from build123d import *

# Parameters (mm, degrees)
F0_R      = 6
F1_DEPTH  = 30
F2_R      = 2.75
F3_DEPTH  = 30.001
F8_R      = 5
F8_R_2    = 1.6
F9_DEPTH  = 2
F12_W     = 4
F12_H     = 30
F13_DEPTH = 3


with BuildPart() as f1:
    # F0 (on Front) → F1 (new body)
    with BuildSketch(Plane.XZ):
        Circle(F0_R)
    extrude(amount=F1_DEPTH)

    # F2 (on face) → F3 (cut, through all)
    with BuildSketch(Plane.XZ.offset(30)):
        Circle(F2_R)
    extrude(amount=-F3_DEPTH, mode=Mode.SUBTRACT)

    # F8 (on face) → F9 (join)
    with BuildSketch(Plane.XZ.offset(30)):
        Circle(F8_R)
        Circle(F8_R_2, mode=Mode.SUBTRACT)
    extrude(amount=-F9_DEPTH)

    # F12 (on offset) → F13 (cut)
    with BuildSketch(Plane.XY.offset(4)):
        with Locations((0, -15)):
            Rectangle(F12_W, F12_H)
    extrude(amount=F13_DEPTH, mode=Mode.SUBTRACT)


solid = f1.part
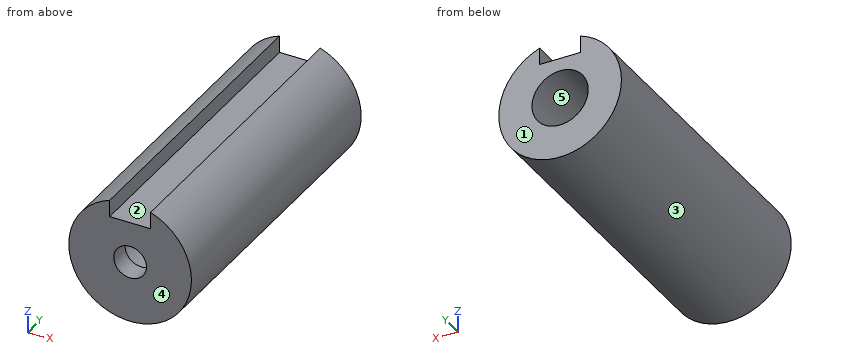
Part model, mm, in its own coordinate system. Face numbers are marked on the shaded views. A direction names the side the tool comes from. Round coordinates to 2 decimals unless told otherwise and drop trailing zeros. Write each loop counter-clockwise with the first axis right and the second up, starting at its lowest first coordinate (ties: lowest second). Pieces come first, ordered by that corner, then holes. Notation, with made-up numbers: M 34,-30.75 L 61,-30.75 A13 ccw 61,-11.75 Z; hole C 20,49 d6. An arc over 180 degrees is marked long. Return JSON: item names as keys, results as strings. Group by question number.
(1) Saw through at A-A on x = 0. Write the cut outline in (y, z), then the cut area to 3 significant figures.
(2) Saw through at B-B on z = 0. Write the cut outline in (x, y), then the cut area to 3 significant figures.
(3) Two-plate mould, pull along X, no slides. Class the marked faces 3, 4 and 5: +X half, -X half, draft (parallel to the pull), parting line (faces both ways), or undercut.
(4) Pin check, flat tips, straight feed: pin 1 Ø0.8 at (y, z) = (-16.5, 4.5) entering from +X; pin 2 Ø1.5 at (y, z) = (-5.5, 3) entering from -X; pin 3 Ø0.5 at (y, z) = (-9.5, 4.5) entering from -X; pin 4 Ø1.9 at (x, z) = (0, 0) entering from +Y. Stop position of each tip, or through.
(5) Which spindle directions (+Z, -Z, +X, -X, +Y, -Y) get a long thin tool onto all of the face, cutting with end or side? Do the marked faces 1 and 2. Say none if no direction does.
(6) Saw through at D-D on x = -3.5. Write the cut outline in (y, z), then the cut area to 3 significant figures.
(7) Drill centre lines: probe 1 along Z at (x, y) = (0, -12.5); probe 2 along Z at (x, y) = (0, -28.5); probe 3 along Y at (x, z) = (1.75, 0). Where is each one in solid material? Low to high.
(8) Saw through at C-C on y = -8.5. Write the cut outline in (x, z), then the cut area to 3 significant figures.
Returned:
{
 "1": {"outline": "M -30,-6 L 0,-6 L 0,-2.75 L -28,-2.75 L -28,-1.6 L -30,-1.6 Z; M -30,1.6 L -28,1.6 L -28,2.75 L 0,2.75 L 0,4 L -30,4 Z", "area": "140 mm²"},
 "2": {"outline": "M -6,-30 L -1.6,-30 L -1.6,-28 L -2.75,-28 L -2.75,0 L -6,0 Z; M 1.6,-30 L 6,-30 L 6,0 L 2.75,0 L 2.75,-28 L 1.6,-28 Z", "area": "200 mm²"},
 "3": {"face 3": "parting line", "face 4": "draft", "face 5": "undercut"},
 "4": {"pin 1": "x = 4.38", "pin 2": "x = -5.56", "pin 3": "x = -4.24", "pin 4": "through"},
 "5": {"face 1": "+Z, -Z, +X, -X, +Y", "face 2": "+Z, +Y, -Y"},
 "6": {"outline": "M -30,-4.87 L 0,-4.87 L 0,4.87 L -30,4.87 Z", "area": "292 mm²"},
 "7": {"probe 1": "-6 to -2.75, 2.75 to 4", "probe 2": "-6 to -1.6, 1.6 to 4", "probe 3": "-30 to -28"},
 "8": {"outline": "M -2,4 L -2,5.66 A6 ccw long 2,5.66 L 2,4 Z; hole C 0,0 d5.5", "area": "81.8 mm²"}
}
